Answer from the drawing. Dimensions are ordinates in mm from the lowest x, y and z of the part. A direction names the side the tool comes from. Give positions to 0.01 mm unless a question says otherwise; leave off trailing zeros. Loops run counter-clockwise (first coordinate to the right, second up) from the corner with the lowest first, then second, coordinate; pieces in that order, holes last. Notation, with made-up numbers: (-5, -23.5) - (46, -23.5) arc R18 cw to (46, -3.5) - close; hole circle Ø3 at (3, 24). An arc over 180 degrees is marked (long way). One line per item, written item: value.
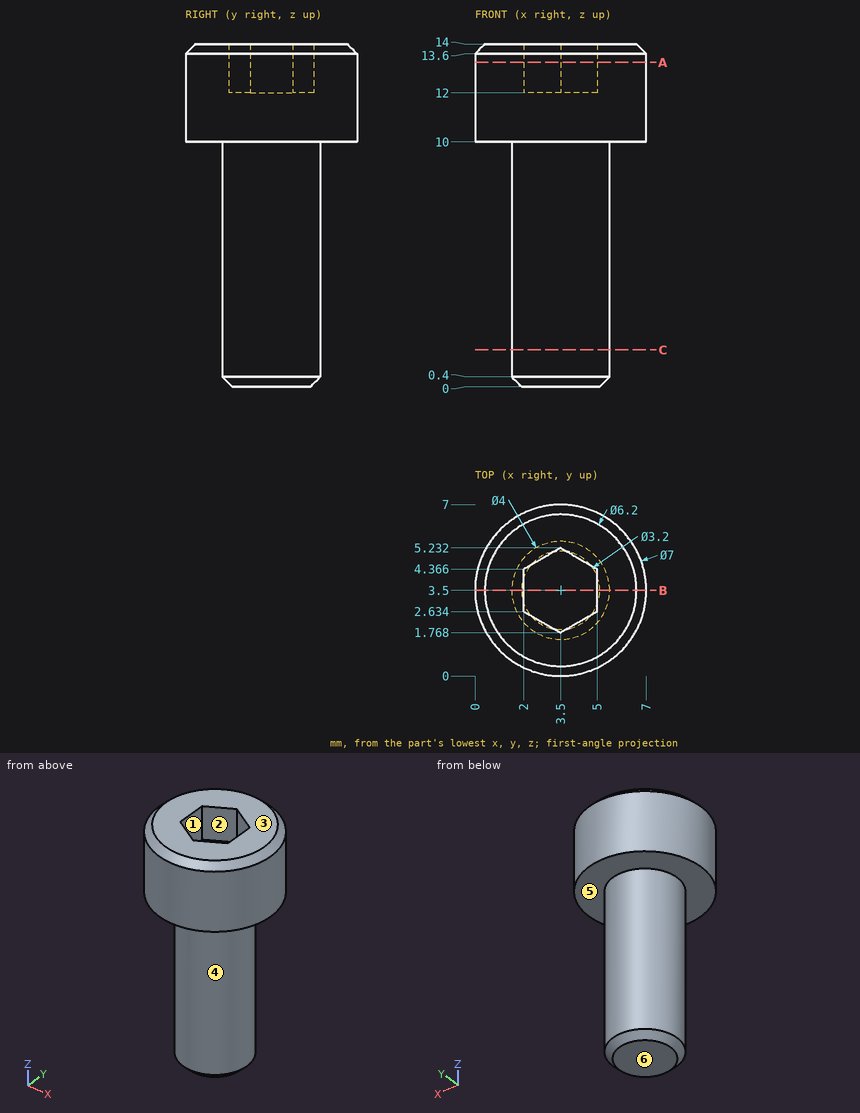
1. The mould has two halves that part along Y. Classify the marked faces 1, 2, 3 and 4: released by +Y, released by -Y, zero draft, split by the parting line, or undercut.
Output:
face 1: undercut
face 2: undercut
face 3: zero draft
face 4: split by the parting line
2. Flat-ended cylindrical pins translate along their axes: pin 1 Ø2 at (x, z) = (1, 6.5) entering from +Y; pin 2 Ø2 at (x, y) = (4, 3) entering from -Z; pin 3 Ø1.5 at (x, z) = (5.5, 8.5) entering from -Y; pin 4 Ø1 at (y, z) = (5, 4.5) entering from +X. Find the tip coordinate at first contact, or state that the pin passes through.
Output:
pin 1: stops at y = 4.82
pin 2: stops at z = 0
pin 3: stops at y = 1.94
pin 4: stops at x = 5.23
3. Section A-A (z = 13.25) is taken. Write down the section's boundary in (x, y), and give its area (3 significant figures).
Output:
outline: circle Ø7 at (3.5, 3.5); hole (2, 2.63) - (3.5, 1.77) - (5, 2.63) - (5, 4.37) - (3.5, 5.23) - (2, 4.37) - close
area: 30.7 mm²
4. Find the intervals of material crossed by line 1 along X through (y, z) = (4.5, 5.75); line 2 along Z through (x, y) = (2, 5.5); line 3 along X through (y, z) = (2, 3.5), in increasing order.
Output:
line 1: x = 1.77 to 5.23
line 2: z = 10 to 14
line 3: x = 2.18 to 4.82
5. Section B-B (y = 3.5) is taken. Write down the section's boundary in (x, z), and give its area (3 significant figures).
Output:
outline: (0, 10) - (1.5, 10) - (1.5, 0.4) - (1.9, 0) - (5.1, 0) - (5.5, 0.4) - (5.5, 10) - (7, 10) - (7, 13.6) - (6.6, 14) - (5, 14) - (5, 12) - (2, 12) - (2, 14) - (0.4, 14) - (0, 13.6) - close
area: 61.7 mm²
6. For the marked faces 5 and 6, determine the directions among +Z, -Z, +X, -X, +Y, -Y from which every point of the face is accessible in a straight line to the end or side of a thin tool.
Output:
face 5: -Z
face 6: -Z, +X, -X, +Y, -Y
7. Section C-C (z = 1.5) is taken. Write down the section's boundary in (x, y).
Output:
outline: circle Ø4 at (3.5, 3.5)
